Input: part model. Units: mm. Frame: model coordinates. Coordinates: 2 decimals unless noted, no trailing zeros. Loops run counter-clockwise (first coordinate to the right, second up) from the corner with the lowest first, then second, coordinate; pieces in that order, holes last.
```python
from build123d import *

# Parameters (mm, degrees)
SKETCH1_R           = 14.2875
SKETCH1_R_2         = 2.5527
SKETCH1_R_3         = 9.525
SKETCH1_R_4         = 3.175
BOSS_EXTRUDE2_DEPTH = 6.35
FILLET1_R           = 6.35


with BuildPart() as part:
    # Sketch1 → Boss-Extrude2 (new body)
    with BuildSketch(Plane.XY):
        with BuildLine():
            Line((-48.689252979, -31.75), (96.8375, -31.75))
            Line((96.8375, -31.75), (96.8375, 22.225))
            Line((96.8375, 22.225), (89.29823289, 54.293104778))
            ThreePointArc((89.29823289, 54.293104778), (78.085476575, 71.830633337), (58.42, 78.654110694))
            Line((58.42, 78.654110694), (-7.62, 78.654110694))
            ThreePointArc((-7.62, 78.654110694), (-27.285476575, 71.830633337), (-38.49823289, 54.293104778))
            Line((-38.49823289, 54.293104778), (-48.689252979, 11.70534681))
            Line((-48.689252979, 11.70534681), (-48.689252979, -31.75))
        make_face()
        Circle(SKETCH1_R, mode=Mode.SUBTRACT)
        with Locations((50.8, 0)):
            Circle(SKETCH1_R, mode=Mode.SUBTRACT)
        with Locations((25.4, 46.904110694)):
            Circle(SKETCH1_R, mode=Mode.SUBTRACT)
        with Locations((-7.62, 72.304110694)):
            Circle(SKETCH1_R_2, mode=Mode.SUBTRACT)
        with Locations((-7.62, 21.504110694)):
            Circle(SKETCH1_R_2, mode=Mode.SUBTRACT)
        with Locations((58.42, 72.304110694)):
            Circle(SKETCH1_R_2, mode=Mode.SUBTRACT)
        with Locations((58.42, 21.504110694)):
            Circle(SKETCH1_R_2, mode=Mode.SUBTRACT)
        with Locations((58.42, 46.904110694)):
            Circle(SKETCH1_R_3, mode=Mode.SUBTRACT)
        with Locations((-7.62, 46.904110694)):
            Circle(SKETCH1_R_3, mode=Mode.SUBTRACT)
        with Locations((75.683179842, 5.09778)):
            Circle(SKETCH1_R_2, mode=Mode.SUBTRACT)
        with Locations((25.916820158, -5.09778)):
            Circle(SKETCH1_R_2, mode=Mode.SUBTRACT)
        with Locations((-41.275, 22.225)):
            Circle(SKETCH1_R_4, mode=Mode.SUBTRACT)
        with Locations((92.075, 22.225)):
            Circle(SKETCH1_R_4, mode=Mode.SUBTRACT)
        with Locations((-41.275, -23.495)):
            Circle(SKETCH1_R_4, mode=Mode.SUBTRACT)
        with Locations((92.075, -23.495)):
            Circle(SKETCH1_R_4, mode=Mode.SUBTRACT)
    extrude(amount=BOSS_EXTRUDE2_DEPTH)

    # Fillet1
    fillet1_edges = [part.edges().sort_by_distance(p)[0] for p in [
        (96.8375, -31.75, 3.175),
        (-48.689252979, -31.75, 3.175),
    ]]
    fillet(fillet1_edges, radius=FILLET1_R)


solid = part.part
```
Item 1: Section query B-B (x = 50.8). Output: boundary loops of the cut face in (y, z).
Result:
outline: (-31.75, 0) - (-14.29, 0) - (-14.29, 6.35) - (-31.75, 6.35) - close; (14.29, 0) - (41.19, 0) - (41.19, 6.35) - (14.29, 6.35) - close; (52.62, 0) - (78.65, 0) - (78.65, 6.35) - (52.62, 6.35) - close
Item 2: Line query: L1, parallel to X at y = 23, z = 4.5; L2, parallel to Y at x = -11, z = 6.25; L3, parallel to X at y = 8, z = 4.25. Output: solid intervals per line, ascending.
Result:
L1: x = -45.99 to -44.35, -38.2 to -9.69, -5.55 to 56.35, 60.49 to 89, 95.15 to 96.66
L2: y = -31.75 to -9.12, 9.12 to 38, 55.81 to 78.47
L3: x = -48.69 to -11.84, 11.84 to 38.96, 62.64 to 96.84
Item 3: Mould query, pull axis X, two halves, no side actions, for faces 1 (the face through (94.93, -29.94, 3.22)), 2 (the face through (-14.274, 0.628, 3.131)), 3 (the face through (23, 24, 0)), 4 (the face through (-48.689, -7, 3)). Classes: +X half, -X half, draft (parallel to the pull), parting line (faces both ways), or undercut.
Result:
face 1: +X half
face 2: undercut
face 3: draft
face 4: -X half
Item 4: Contact query for flat-ended pins moving along their axis: P1, Ø1.5, axis at y = 49.5, z = 1, coming from the -X side; P2, Ø1.5, axis at y = 58.5, z = 4.5, coming from the -X side. Output: stop coordinate, or through.
Result:
P1: stops at x = -39.82
P2: stops at x = -37.46
Item 5: Section query C-C (z = 4.5). Count the separate pieces of the cut face and the enclosed holes in it, then the cut area to 3 significant figures.
Result:
separate pieces: 1
enclosed holes: 15
area: 12,200 mm2
Item 6: Section query D-D (x = 80.5). Output: boundary loops of the cut face in (y, z), then the cut area to 3 significant figures.
Result:
outline: (-31.75, 0) - (69.72, 0) - (69.72, 6.35) - (-31.75, 6.35) - close
area: 644 mm2
Item 7: Section query A-A (y = 0). Output: boundary loops of the cut face in (x, z).
Result:
outline: (-48.69, 0) - (-14.29, 0) - (-14.29, 6.35) - (-48.69, 6.35) - close; (14.29, 0) - (36.51, 0) - (36.51, 6.35) - (14.29, 6.35) - close; (65.09, 0) - (96.84, 0) - (96.84, 6.35) - (65.09, 6.35) - close
